Verification items for the finished model (mm, model axes). Coordinates: 2 decimals unless noted, no trailing zeros. Order: outer loops, then holes, each group sorted by start corner. A loop starts at its lowest first (then second) coordinate and runs counter-clockwise, first axis right, second up.
Q1. Draft check along Z on faces 1 (the flat face through (-2, 3, 101.6)), 2 (the cylindrical face through (-2.4, 3.1, 4.5)), 3 (the flat face through (-2, 0, -24)), 4 (the flat face through (-2, 3, -101.6)). Enter one of: pulls with the +Z half, pulls with the -Z half, needs draft (parallel to the pull), parting line crosses it, or undercut.
Q2. Cross-section at A-A, the plane z = 0. Record the boundary of the cut face in (x, y), and give its area (3 significant figures).
Q3. Thickness scan on line 1 (X direction, y = 1.5, z = -81.28); line 2 (Z direction, x = 1, y = 5.25); line 3 (X direction, y = 4.5, z = -3). Record the ranges inside material, lowest first.
from build123d import *

# Parameters (mm, degrees)
SKETCH2_W                         = 355.6
SKETCH2_H                         = 203.2
BOSS_EXTRUDE1_DEPTH               = 6.35
SKETCH3_R                         = 2.54
CUT_EXTRUDE1_DEPTH                = 205.879775722
TAP_DRILL_FOR_M12X1_75_TAP1_D     = 10.2
TAP_DRILL_FOR_M12X1_75_TAP1_DEPTH = 19.05
TAP_DRILL_FOR_M12X1_75_TAP1_TIP   = 3.064389157


with BuildPart() as part:
    # Sketch2 → Boss-Extrude1 (new body)
    with BuildSketch(Plane(origin=(0, 0, 0), x_dir=(1, 0, 0), z_dir=(0, 1, 0))):
        Rectangle(SKETCH2_W, SKETCH2_H)
    extrude(amount=BOSS_EXTRUDE1_DEPTH)

    # Sketch3 → Cut-Extrude1 (cut, through all)
    with BuildSketch(Plane(origin=(0, 6.35, 0), x_dir=(1, 0, 0), z_dir=(0, 1, 0))):
        with Locations(Location((0, 81.28, 0), (0, 0, 270))):
            Circle(SKETCH3_R)
        with Locations(Location((0, 60.779914, 0), (0, 0, 270))):
            Circle(SKETCH3_R)
    extrude(amount=-CUT_EXTRUDE1_DEPTH, mode=Mode.SUBTRACT)

    # Tap Drill for M12x1.75 Tap1
    with Locations(Plane(origin=(0, 6.35, 0), x_dir=(1, 0, 0), z_dir=(0, 1, 0))):
        with Locations((0, 0)):
            Hole(TAP_DRILL_FOR_M12X1_75_TAP1_D / 2, depth=TAP_DRILL_FOR_M12X1_75_TAP1_DEPTH)
            with Locations((0, 0, -(TAP_DRILL_FOR_M12X1_75_TAP1_DEPTH + TAP_DRILL_FOR_M12X1_75_TAP1_TIP / 2))):  # 118° drill point
                Cone(0, TAP_DRILL_FOR_M12X1_75_TAP1_D / 2, TAP_DRILL_FOR_M12X1_75_TAP1_TIP, mode=Mode.SUBTRACT)


solid = part.part
Check values:
1. face 1: pulls with the +Z half
1. face 2: undercut
1. face 3: needs draft
1. face 4: pulls with the -Z half
2. outline: (-177.8, 0) - (-5.1, 0) - (-5.1, 6.35) - (-177.8, 6.35) - close; (5.1, 0) - (177.8, 0) - (177.8, 6.35) - (5.1, 6.35) - close
2. area: 2,190 mm2
3. line 1: x = -177.8 to -2.54, 2.54 to 177.8
3. line 2: z = -101.6 to -83.61, -78.95 to -63.11, -58.45 to -5, 5 to 101.6
3. line 3: x = -177.8 to -4.12, 4.12 to 177.8
